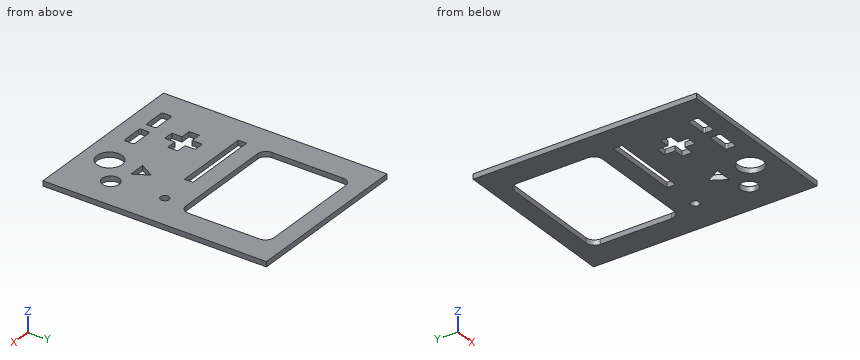
from build123d import *

# Parameters (mm, degrees)
SKETCH1_W           = 101
SKETCH1_H           = 132
BOSS_EXTRUDE1_DEPTH = 1.5
SKETCH2_R           = 7.5
SKETCH2_R_2         = 5
SKETCH2_R_3         = 2.5
SKETCH2_W           = 45
SKETCH2_H           = 5
CUT_EXTRUDE2_DEPTH  = 84.157982179


with BuildPart() as part:
    # Sketch1 → Boss-Extrude1 (new, symmetric)
    with BuildSketch(Plane.XY):
        Rectangle(SKETCH1_W, SKETCH1_H)
    extrude(amount=BOSS_EXTRUDE1_DEPTH, both=True)

    # Sketch2 → Cut-Extrude2 (cut, through all)
    with BuildSketch(Plane.XY.offset(1.5)):
        with Locations((16, -51)):
            Circle(SKETCH2_R)
        with Locations((32, -39)):
            Circle(SKETCH2_R_2)
        with Locations((30, -8.5)):
            Circle(SKETCH2_R_3)
        with BuildLine():
            Line((-30, 4), (30, 4))
            ThreePointArc((30, 4), (33.535533906, 5.464466094), (35, 9))
            Line((35, 9), (35, 51))
            ThreePointArc((35, 51), (33.535533906, 54.535533906), (30, 56))
            Line((30, 56), (-30, 56))
            ThreePointArc((-30, 56), (-33.535533906, 54.535533906), (-35, 51))
            Line((-35, 51), (-35, 9))
            ThreePointArc((-35, 9), (-33.535533906, 5.464466094), (-30, 4))
        make_face()
        Polygon((11, -35), (21, -35), (16, -26.339745962), align=None)
        with BuildLine():
            Line((-15.5, -56), (-4, -56))
            ThreePointArc((-4, -56), (-3.292893219, -55.707106781), (-3, -55))
            Line((-3, -55), (-3, -51))
            ThreePointArc((-3, -51), (-3.292893219, -50.292893219), (-4, -50))
            Line((-4, -50), (-15.5, -50))
            ThreePointArc((-15.5, -50), (-16.207106781, -50.292893219), (-16.5, -51))
            Line((-16.5, -51), (-16.5, -55))
            ThreePointArc((-16.5, -55), (-16.207106781, -55.707106781), (-15.5, -56))
        make_face()
        with BuildLine():
            Line((-34, -56), (-22.5, -56))
            ThreePointArc((-22.5, -56), (-21.792893219, -55.707106781), (-21.5, -55))
            Line((-21.5, -55), (-21.5, -51))
            ThreePointArc((-21.5, -51), (-21.792893219, -50.292893219), (-22.5, -50))
            Line((-22.5, -50), (-34, -50))
            ThreePointArc((-34, -50), (-34.707106781, -50.292893219), (-35, -51))
            Line((-35, -51), (-35, -55))
            ThreePointArc((-35, -55), (-34.707106781, -55.707106781), (-34, -56))
        make_face()
        Polygon((-22, -41), (-16, -41), (-16, -35), (-10, -35), (-10, -29), (-16, -29), (-16, -23), (-22, -23), (-22, -29), (-28, -29), (-28, -35), (-22, -35), align=None)
        with Locations((-12.5, -8.5)):
            Rectangle(SKETCH2_W, SKETCH2_H)
    extrude(amount=-CUT_EXTRUDE2_DEPTH, mode=Mode.SUBTRACT)


solid = part.part
Input: part model. Units: mm. Frame: model coordinates. Coordinates: 2 decimals unless noted, no trailing zeros. Loops run counter-clockwise (first coordinate to the right, second up) from the corner with the lowest first, then second, coordinate; pieces in that order, holes last.
(1) Section D-D on z = -0.1. Count the separate pieces of the cut face and the enclosed holes in it, then the cut area to 3 significant figures.
(2) Section B-B on x = 2. Return the cut outline in (y, z), then the cut area to 3 significant figures.
(3) Section C-C on y = 22. Return the cut outline in (x, z), then the cut area to 3 significant figures.
(4) Section A-A on y = -8.5. Return the cut outline in (x, z).
(5) Material intervals for probe 1 along Y at (x, z) = (-15, 0.35); probe 2 along X at (y, z) = (33, -0.3); probe 3 along Y at (x, z) = (9.5, 0), sorted ascending.
Data:
1. separate pieces: 1
1. enclosed holes: 9
1. area: 8,830 mm2
2. outline: (-66, -1.5) - (-11, -1.5) - (-11, 1.5) - (-66, 1.5) - close; (-6, -1.5) - (4, -1.5) - (4, 1.5) - (-6, 1.5) - close; (56, -1.5) - (66, -1.5) - (66, 1.5) - (56, 1.5) - close
2. area: 225 mm2
3. outline: (-50.5, -1.5) - (-35, -1.5) - (-35, 1.5) - (-50.5, 1.5) - close; (35, -1.5) - (50.5, -1.5) - (50.5, 1.5) - (35, 1.5) - close
3. area: 93.0 mm2
4. outline: (-50.5, -1.5) - (-35, -1.5) - (-35, 1.5) - (-50.5, 1.5) - close; (10, -1.5) - (27.5, -1.5) - (27.5, 1.5) - (10, 1.5) - close; (32.5, -1.5) - (50.5, -1.5) - (50.5, 1.5) - (32.5, 1.5) - close
5. probe 1: y = -66 to -56, -50 to -35, -29 to -11, -6 to 4, 56 to 66
5. probe 2: x = -50.5 to -35, 35 to 50.5
5. probe 3: y = -66 to -54.74, -47.26 to -11, -6 to 4, 56 to 66
